Can you work these out from the model? Positions are in its coordinate system, mm. A direction names the side the tool comes from. Give positions to 0.01 mm unless a question says otherwise; leave off trailing zeros. Write each loop counter-clockwise with the first axis right and the second up, starting at its lowest first coordinate (ties: lowest second). Pieces come first, ordered by that corner, then holes.
from build123d import *

# Parameters (mm, degrees)
F1_DEPTH = 5
F3_DEPTH = 10
F4_R     = 1


# Not quite as in the source:
# - a feature names something its author has since deleted; it is built from what else it names


with BuildPart() as f1:
    # F0 (on Top) → F1 (new body)
    with BuildSketch(Plane.XY):
        with BuildLine():
            Line((29, -41.5), (29, 41.5))
            ThreePointArc((29, 41.5), (26.5104076401, 47.5104076401), (20.5, 50))
            Line((20.5, 50), (-20.5, 50))
            ThreePointArc((-20.5, 50), (-26.5104076401, 47.5104076401), (-29, 41.5))
            Line((-29, 41.5), (-29, -41.5))
            ThreePointArc((-29, -41.5), (-26.5104076401, -47.5104076401), (-20.5, -50))
            Line((-20.5, -50), (20.5, -50))
            ThreePointArc((20.5, -50), (26.5104076401, -47.5104076401), (29, -41.5))
        make_face()
    extrude(amount=F1_DEPTH)

    # F2 (on Top) → F3 (join)
    with BuildSketch(Plane.XY):
        with BuildLine():
            ThreePointArc((32.5, 41.5), (28.9852813742, 49.9852813742), (20.5, 53.5))
            Line((20.5, 53.5), (-20.5, 53.5))
            ThreePointArc((-20.5, 53.5), (-28.9852813742, 49.9852813742), (-32.5, 41.5))
            Line((-32.5, 41.5), (-32.5, -41.5))
            ThreePointArc((-32.5, -41.5), (-28.9852813742, -49.9852813742), (-20.5, -53.5))
            Line((-20.5, -53.5), (20.5, -53.5))
            ThreePointArc((20.5, -53.5), (28.9852813742, -49.9852813742), (32.5, -41.5))
            Line((32.5, -41.5), (32.5, 41.5))
        make_face()
    extrude(amount=-F3_DEPTH)

    # F4
    f4_edges = [f1.edges().sort_by_distance(p)[0] for p in [
        (0, 50, 5),
        (-26.510408, 47.510408, 5),
        (-29, 0, 5),
        (-26.510408, -47.510408, 5),
        (0, -50, 5),
        (26.510408, -47.510408, 5),
        (29, 0, 5),
        (26.510408, 47.510408, 5),
    ]]
    fillet(f4_edges, radius=F4_R)


solid = f1.part
(1) For faces 1 (the face through (0, 50, 2)), 2 (the face through (26.44, -47.58, 1.97)), 3 (the face through (26.58, 47.44, 1.97)), 4 (the face through (-26.58, -47.44, 1.97)), 5 (the face through (0, -50, 2)), which set-ups out of +Z, -Z, +X, -X, +Y, -Y let a thin tool reach every point of the face, with its end or its side?
Returned:
face 1: +Z, +X, -X, +Y
face 2: +Z, +X, -Y
face 3: +Z, +X, +Y
face 4: +Z, -X, -Y
face 5: +Z, +X, -X, -Y
(2) Imagine slicing it at B-B, the plane z = -1.75. Write out the boundary of the cut face in (x, y).
Returned:
outline: (-32.5, -41.5) arc R12 ccw to (-20.5, -53.5) - (20.5, -53.5) arc R12 ccw to (32.5, -41.5) - (32.5, 41.5) arc R12 ccw to (20.5, 53.5) - (-20.5, 53.5) arc R12 ccw to (-32.5, 41.5) - close
(3) Imagine slicing it at A-A, the plane y = -34.5. Write out the boundary of the cut face in (x, z).
Returned:
outline: (-32.5, -10) - (32.5, -10) - (32.5, 0) - (29, 0) - (29, 4) arc R1 ccw to (28, 5) - (-28, 5) arc R1 ccw to (-29, 4) - (-29, 0) - (-32.5, 0) - close
(4) If I drill on L1, parallel to X at y = -7, z = 0.25; L2, parallel to Y at x = -17, z = 1; L3, parallel to Z at x = 30, y = -29, over which ranges is the centre line in solid material (lowest first)?
Returned:
L1: x = -29 to 29
L2: y = -50 to 50
L3: z = -10 to 0
(5) Imagine slicing it at C-C, the plane x = 11. Write out the boundary of the cut face in (y, z).
Returned:
outline: (-53.5, -10) - (53.5, -10) - (53.5, 0) - (50, 0) - (50, 4) arc R1 ccw to (49, 5) - (-49, 5) arc R1 ccw to (-50, 4) - (-50, 0) - (-53.5, 0) - close
(6) Will these pins go through, and if not, where does the flat tip stop? P1, Ø1.2, axis at x = -8.5, z = 1.5, coming from the +Y side; P2, Ø2, axis at y = -19, z = 2, coming from the +X side; P3, Ø4, axis at x = -23, z = 1.5, coming from the -Y side; P4, Ø5, axis at x = 22, z = -1, coming from the -Y side.
Returned:
P1: stops at y = 50
P2: stops at x = 29
P3: stops at y = -53.44
P4: stops at y = -53.5
